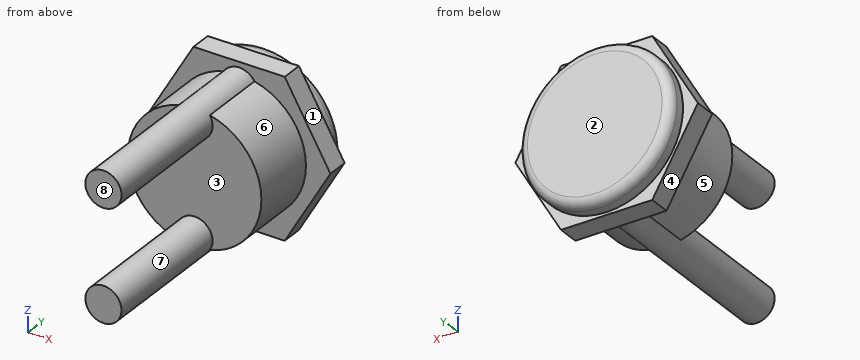
from build123d import *

# Parameters (mm, degrees)
SKETCH1_R           = 10.7315
BOSS_EXTRUDE1_DEPTH = 2.54
BOSS_EXTRUDE2_DEPTH = 3.048
SKETCH4_R           = 9.398
BOSS_EXTRUDE4_DEPTH = 9.525
SKETCH3_R           = 2.54
BOSS_EXTRUDE3_DEPTH = 29
FILLET1_R           = 1.27


with BuildPart() as part:
    # Sketch1 → Boss-Extrude1 (new body)
    with BuildSketch(Plane(origin=(0, 0, 0), x_dir=(1, 0, 0), z_dir=(0, 1, 0))):
        with Locations(Location((0, 0, 0), (0, 0, 270))):
            Circle(SKETCH1_R)
    extrude(amount=BOSS_EXTRUDE1_DEPTH)

    # Sketch2 → Boss-Extrude2 (add)
    with BuildSketch(Plane.XZ):
        Polygon((-12.831609733, 0), (-6.415804866, -11.1125), (6.415804866, -11.1125), (12.831609733, 0), (6.415804866, 11.1125), (-6.415804866, 11.1125), align=None)
    extrude(amount=BOSS_EXTRUDE2_DEPTH)

    # Sketch4 → Boss-Extrude4 (add)
    with BuildSketch(Plane.XZ.offset(3.048)):
        with Locations(Location((0, 0, 0), (0, 0, 90))):
            Circle(SKETCH4_R)
    extrude(amount=BOSS_EXTRUDE4_DEPTH)

    # Sketch3 → Boss-Extrude3 (add)
    with BuildSketch(Plane.XZ.offset(3.048)):
        with Locations(Location((0, 7.80660503, 0), (0, 0, 31.85091732))):
            Circle(SKETCH3_R)
        with Locations(Location((0, -7.80660503, 0), (0, 0, 211.85091732))):
            Circle(SKETCH3_R)
    extrude(amount=BOSS_EXTRUDE3_DEPTH)

    # Fillet1
    fillet1_edges = [part.edges().sort_by_distance(p)[0] for p in [
        (0, 2.54, -10.7315),
    ]]
    fillet(fillet1_edges, radius=FILLET1_R)


solid = part.part
Work out the finished part from the listing and answer in its coordinate system (mm). Face numbers are marked on the shaded views. A direction names the side the tool comes from. Round coordinates to 2 decimals unless told otherwise and drop trailing zeros. Write each loop counter-clockwise with the first axis right and the second up, starting at its lowest first coordinate (ties: lowest second). Pieces come first, ordered by that corner, then holes.
1) Straight lines are drawn through the part: line 1 (Z direction, x = 0, y = -20.5); line 2 (Y direction, x = -3.5, z = 6.5); line 3 (Y direction, x = 3.5, z = -9.75). For each, find the intervals that lie inside material, in ascending order.
2) A cutting plane is placed at A-A (x = 0). Give the vertices of the cut face in (y, z).
3) Given pin 1 Ø1 at (x, z) = (-2.5, 6) entering from -Y; pin 2 Ø12 at (x, y) = (3, -13) entering from +Z; pin 3 Ø1 at (y, z) = (-11, 8) entering from +X, each flat-ended and moving along its own axis, determine where each tip first touches the part or whether it passes through.
4) A tool of negligible diameter and unlimited length cuts with its end or side. For the marked faces 4, 5, 6, 7 and 8, from which of +Z, -Z, +X, -X, +Y, -Y can it reach the whole face along a straight path? Write none if from no direction.
5) The mould has two halves that part along Z. Classify the marked faces 1, 2 and 3: pulls with the +Z half, pulls with the -Z half, needs draft (parallel to the pull), parting line crosses it, or undercut.
6) A cutting plane is placed at B-B (y = -13). Give the vertices of the cut face in (x, z).
Completed:
1. line 1: z = -10.35 to -5.27, 5.27 to 10.35
1. line 2: y = -12.57 to 2.54
1. line 3: y = -3.05 to 2.17
2. outline: (-32.05, -10.35) - (-3.05, -10.35) - (-3.05, -11.11) - (0, -11.11) - (0, -10.73) - (1.27, -10.73) arc R1.27 ccw to (2.54, -9.46) - (2.54, 9.46) arc R1.27 ccw to (1.27, 10.73) - (0, 10.73) - (0, 11.11) - (-3.05, 11.11) - (-3.05, 10.35) - (-32.05, 10.35) - (-32.05, 5.27) - (-12.57, 5.27) - (-12.57, -5.27) - (-32.05, -5.27) - close
3. pin 1: stops at y = -12.57
3. pin 2: stops at z = 10.35
3. pin 3: stops at x = 5.66
4. face 4: -Z, -X, +Y, -Y
4. face 5: -X, -Y
4. face 6: +X, -Y
4. face 7: -Y
4. face 8: +Z, -Z, +X, -X, -Y
5. face 1: pulls with the +Z half
5. face 2: needs draft
5. face 3: undercut
6. outline: circle Ø5.08 at (0, -7.81); circle Ø5.08 at (0, 7.81)
